Input: part model. Units: mm. Frame: model coordinates. A direction names the side the tool comes from. Give positions to 0.01 mm unless a question says otherwise; leave off trailing zeros. Order: outer loops, then holes, each group sorted by start corner. A loop starts at its lowest first (then second) coordinate and runs counter-clockwise, first axis right, second up. Notation, with made-up numbers: (24, 59.5) - (47, 59.5) arc R26 cw to (47, 97.5) - close; hole circle Ø8 at (54, 47.25). An arc over 180 degrees is marked (long way). Answer in a Markdown table with one row per item. Add a question column.
1. Section query C-C on y = 0. Return loops of the section in (x, z).
2. Mould query, pull axis Y, two halves, no side actions, for faces 6 (the face through (-18.015, 0.7, 8.2)), 7 (the face through (1, 0, 5)), 8 (the face through (-27.01, 0.38, 17.48)). Classes: released by +Y, released by -Y, zero draft, split by the parting line, or undercut.
3. Contact query for flat-ended pins moving along their axis: pin 1 (10 mm diameter, centred on y = -27, z = 23, fed in from +X); pin 2 (12 mm diameter, centred on x = -17, z = 12, fed in from +Y); pin 3 (8 mm diameter, centred on y = -21, z = 11.5, fed in from -X). Output: stop coordinate, or through.
4. Section query D-D on x = 29.5. Return loops of the section in (y, z), and give its area (3 significant figures).
5. Access query for faces 1 (the face through (12.257, -0.7, 8.2)), 2 (the face through (38.592, 0.209, 9.498)), 3 (the face through (-36.084, 0.572, 25.994)), 4 (the face through (50, 0, 6)), 5 (the face through (-11.3, 7.8, 0)). Directions: +Z, -Z, +X, -X, +Y, -Y. A direction counts if a zero-diameter tool reaches every point of the face in a straight line with its end or side. Return the directions, or none.
6. Section query A-A on z = 22.5. Return loops of the section in (x, y), and give its area (3 significant figures).
7. Ray query, line 1 (X direction, y = -10, z = 17.5); line 2 (X direction, y = 0, z = 17); line 3 (X direction, y = -12, z = 31.5). Return the intervals inside material, ascending. Write a range as [from, to].
8. Section query B-B on y = 21.5. Return loops of the section in (x, z).
```python
from build123d import *

# Parameters (mm, degrees)
REVOLUTION_ANGLE   = 180
SKETCH001_R        = 2.5
POCKET_DEPTH       = 22
POLARPATTERN_COUNT = 12


with BuildPart() as part:
    # Sketch → Revolution (revolve)
    with BuildSketch(Plane.XY):
        Polygon((27.5, 9.5), (27.5, 17.46), (20.5, 17.46), (20.5, 18.46), (20, 18.46), (20, 24), (17.5, 24), (17.5, 13.242641), (16.5, 13.242641), (12.257359, 9), (12.257359, 8), (-18.014719, 8), (-18.014719, 9), (-26.5, 17.485281), (-27.5, 17.485281), (-27.5, 34), (-30, 34), (-30, 26), (-42, 26), (-42, 9.5), (-50, 9.5), (-50, 5), (50, 5), (50, 9.5), align=None)
    revolve(axis=Axis((0, 0, 0), (1, 0, 0)), revolution_arc=REVOLUTION_ANGLE)

    # Sketch001 → Pocket (cut)
    with BuildSketch(Plane(origin=(-74.5, 0, 0), x_dir=(0, -1, 0), z_dir=(-1, 0, 0))):
        with Locations((0, 22)):
            Circle(SKETCH001_R)
        with Locations((0, 15)):
            Circle(SKETCH001_R)
    pocket = extrude(amount=-POCKET_DEPTH, mode=Mode.SUBTRACT)

    # PolarPattern: Pocket ×12 about axis
    polarpattern_axis = Axis((-74.5, 0, 0), (-1, 0, 0))
    for i in range(1, POLARPATTERN_COUNT):
        add(pocket.rotate(polarpattern_axis, i * 360 / POLARPATTERN_COUNT), mode=Mode.SUBTRACT)


solid = part.part
```
Answer:
| question | item | result |
|---|---|---|
| 1 | outline | (-50, 5) - (50, 5) - (50, 9.5) - (27.5, 9.5) - (27.5, 17.46) - (20.5, 17.46) - (20.5, 18.46) - (20, 18.46) - (20, 24) - (17.5, 24) - (17.5, 13.24) - (16.5, 13.24) - (12.26, 9) - (12.26, 8) - (-18.01, 8) - (-18.01, 9) - (-26.5, 17.49) - (-27.5, 17.49) - (-27.5, 34) - (-30, 34) - (-30, 26) - (-42, 26) - (-42, 9.5) - (-50, 9.5) - close |
| 2 | face 6 | zero draft |
| 2 | face 7 | undercut |
| 2 | face 8 | split by the parting line |
| 3 | pin 1 | stops at x = -27.5 |
| 3 | pin 2 | stops at y = 9.65 |
| 3 | pin 3 | stops at x = -42 |
| 4 | outline | (-9.5, 0) - (-5, 0) arc R5 cw to (5, 0) - (9.5, 0) arc R9.5 ccw to start |
| 4 | area | 102 mm² |
| 5 | face 1 | +Z |
| 5 | face 2 | +Z, +X |
| 5 | face 3 | +Z, -X |
| 5 | face 4 | +Z, -Z, +X, +Y, -Y |
| 5 | face 5 | -Z, +X, -X, +Y, -Y |
| 6 | outline | (-42, -13.03) - (-30, -13.03) - (-30, -25.49) - (-27.5, -25.49) - (-27.5, 25.49) - (-30, 25.49) - (-30, 13.03) - (-42, 13.03) - close; (17.5, -8.35) - (20, -8.35) - (20, 8.35) - (17.5, 8.35) - close |
| 6 | area | 482 mm² |
| 7 | line 1 | x = [-42, -27.5], [17.5, 20] |
| 7 | line 2 | x = [-42, -26.01], [17.5, 27.5] |
| 7 | line 3 | x = [-30, -27.5] |
| 8 | outline | (-42, 0) - (-27.5, 0) - (-27.5, 26.34) - (-30, 26.34) - (-30, 14.62) - (-42, 14.62) - close; (17.5, 0) - (20, 0) - (20, 10.67) - (17.5, 10.67) - close |
